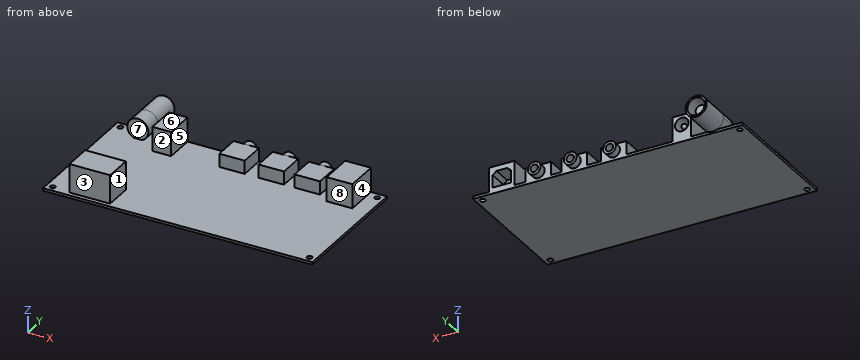
from build123d import *

# Parameters (mm, degrees)
F0_W           = 127
F0_H           = 63
F1_DEPTH       = 1.2
F2_R           = 1.25
F3_DEPTH       = 1.2
F4_W           = 12
F4_H           = 12.13
F5_DEPTH       = 6.25
F6_R           = 3
F7_DEPTH       = 3.52
F8_R           = 1.775
F9_DEPTH       = 14
F10_W          = 12.12
F10_H          = 15.7
F11_DEPTH      = 11.43
F13_DEPTH      = 9
F14_W          = 8.84
F14_H          = 13.9
F15_DEPTH      = 11.4
F16_R          = 3.2
F17_DEPTH      = 9.25
F18_R          = 1.15
F19_DEPTH      = 8.25
F20_R          = 1
F21_R          = 5
F22_DEPTH      = 14
F22_DEPTH_BACK = 8
F23_R          = 4.1
F24_DEPTH      = 8.6
F25_R          = 2.3
F26_DEPTH      = 4.9
F27_W          = 19.16
F27_H          = 13.3
F28_DEPTH      = 13.46


with BuildPart() as f1:
    # F0 (on Top) → F1 (new body)
    with BuildSketch(Plane.XY):
        with Locations((63.5, -31.5)):
            Rectangle(F0_W, F0_H)
    extrude(amount=F1_DEPTH)

    # F2 (on face) → F3 (cut, through all)
    with BuildSketch(Plane.XY.offset(1.2)):
        with Locations((2.955, -2.955)):
            Circle(F2_R)
        with Locations((2.955, -60.045)):
            Circle(F2_R)
        with Locations((124.045, -60.045)):
            Circle(F2_R)
        with Locations((124.045, -2.955)):
            Circle(F2_R)
    extrude(amount=-F3_DEPTH, mode=Mode.SUBTRACT)

    # F4 (on face) → F5 (join)
    with BuildSketch(Plane.XY.offset(1.2)):
        with Locations((96.19, -6.065)):
            Rectangle(F4_W, F4_H)
        with Locations((79.2, -6.065)):
            Rectangle(F4_W, F4_H)
        with Locations((60.7, -6.065)):
            Rectangle(F4_W, F4_H)
    extrude(amount=F5_DEPTH)

    # F6 (on face) → F7 (join)
    with BuildSketch(Plane(origin=(0, 0, 0), x_dir=(-1, 0, 0), z_dir=(0, 1, 0))):
        with Locations((-96.19, 4.325)):
            Circle(F6_R)
        with Locations((-79.2, 4.325)):
            Circle(F6_R)
        with Locations((-60.7, 4.325)):
            Circle(F6_R)
    extrude(amount=F7_DEPTH)

    # F8 (on face) → F9 (cut)
    with BuildSketch(Plane(origin=(0, 3.52, 0), x_dir=(-1, 0, 0), z_dir=(0, 1, 0))):
        with Locations((-96.19, 4.325)):
            Circle(F8_R)
        with Locations((-79.2, 4.325)):
            Circle(F8_R)
        with Locations((-60.7, 4.325)):
            Circle(F8_R)
    extrude(amount=-F9_DEPTH, mode=Mode.SUBTRACT)

    # F10 (on face) → F11 (join)
    with BuildSketch(Plane.XY.offset(1.2)):
        with Locations((113.39, -7.85)):
            Rectangle(F10_W, F10_H)
    extrude(amount=F11_DEPTH)

    # F12 (on face) → F13 (cut)
    with BuildSketch(Plane(origin=(0, 0, 0), x_dir=(-1, 0, 0), z_dir=(0, 1, 0))):
        Polygon((-117.78, 8.72), (-117.78, 2.8), (-109, 2.8), (-109, 8.72), (-110.89, 10.2), (-115.89, 10.2), align=None)
    extrude(amount=-F13_DEPTH, mode=Mode.SUBTRACT)

    # F14 (on face) → F15 (join)
    with BuildSketch(Plane.XY.offset(1.2)):
        with Locations((28.58, -6.95)):
            Rectangle(F14_W, F14_H)
    extrude(amount=F15_DEPTH)

    # F16 (on face) → F17 (cut)
    with BuildSketch(Plane(origin=(0, 0, 0), x_dir=(-1, 0, 0), z_dir=(0, 1, 0))):
        with Locations((-28.58, 8.1)):
            Circle(F16_R)
    extrude(amount=-F17_DEPTH, mode=Mode.SUBTRACT)

    # F18 (on face) → F19 (join, through all)
    with BuildSketch(Plane(origin=(0, -9.25, 0), x_dir=(-1, 0, 0), z_dir=(0, 1, 0))):
        with Locations((-28.58, 8.1)):
            Circle(F18_R)
    extrude(amount=F19_DEPTH)

    # F20
    f20_edges = [f1.edges().sort_by_distance(p)[0] for p in [
        (29.73, -1, 8.1),
    ]]
    fillet(f20_edges, radius=F20_R)

    # F21 (on face) → F22 (join, two sides)
    with BuildSketch(Plane(origin=(0, 0, 0), x_dir=(-1, 0, 0), z_dir=(0, 1, 0))) as f22_sk:
        with Locations((-14, 5.77)):
            Circle(F21_R)
    extrude(amount=F22_DEPTH)
    extrude(f22_sk.sketch, amount=-F22_DEPTH_BACK)

    # F23 (on face) → F24 (cut)
    with BuildSketch(Plane(origin=(0, 14, 0), x_dir=(-1, 0, 0), z_dir=(0, 1, 0))):
        with Locations((-14, 5.77)):
            Circle(F23_R)
    extrude(amount=-F24_DEPTH, mode=Mode.SUBTRACT)

    # F25 (on face) → F26 (join, through all)
    with BuildSketch(Plane(origin=(0, 5.4, 0), x_dir=(-1, 0, 0), z_dir=(0, 1, 0))):
        with Locations((-14, 5.77)):
            Circle(F25_R)
    extrude(amount=F26_DEPTH)

    # F27 (on face) → F28 (join)
    with BuildSketch(Plane.XY.offset(1.2)):
        with Locations((20.88, -54.24)):
            Rectangle(F27_W, F27_H)
    extrude(amount=F28_DEPTH)


solid = f1.part
The listing builds one solid part. Answer for the finished solid, in the listing's coordinates (mm). Face numbers are marked on the shaded views. A direction names the side the tool comes from. Coordinates: 2 decimals unless noted, no trailing zeros. Write each loop counter-clockwise with the first axis right and the second up, starting at its lowest first coordinate (ties: lowest second). Pieces come first, ordered by that corner, then holes. Notation, with made-up numbers: M -13.75,73.25 L 4.25,73.25 A17 ccw 4.25,99.25 Z; hole C -22,15 d4. An arc over 180 degrees is marked long. Put each result on its own line as item: value. Start each with the question number.
1. A cutting plane is placed at C-C on x = 79.2. Write down the section's boundary in (y, z) (3 decimals).
2. A cutting plane is placed at A-A on y = -54. Write down the section's boundary in (x, z), then the cut area to 3 significant figures.
3. For a pull along Y with two mould halves and no side action, classify the marked faces 6, 7 and 8 as pulls with the +Y half, pulls with the -Y half, needs draft (parallel to the pull), parting line crosses it, or undercut.
4. A cutting plane is placed at B-B on x = 14. Write down the section's boundary in (y, z), then the cut area to 3 significant figures.
5. Which of the six approach directions +Z, -Z, +X, -X, +Y, -Y give full straight-line access (tool end or side, diameter ignored) to the marked faces 1, 2, 3, 4 and 5?
6. Consider line 1 (Z direction, x = 14, y = 8); line 2 (X direction, y = -7, z = 1.25); line 3 (Z direction, x = 96, y = -3). Determine where each line is inside the solid, lowest interval first. Write a range as from..to.
7. A cutting plane is placed at D-D on y = -40.5. Write down the section's boundary in (x, z).
8. Flat-ended cylindrical pins translate along their axes: P1, Ø1.9, axis at x = 58.5, z = 3.5, coming from the -Y side; P2, Ø8, axis at x = 50.5, z = 2.5, coming from the +Y side; P3, Ø1.8, axis at x = 80, z = 3.5, coming from the +Y side. Find the tip coordinate at first contact, or state that the pin passes through.
Resolved:
1. outline: M -63,0 L 0,0 L 0,1.325 L 3.52,1.325 L 3.52,2.55 L -10.48,2.55 L -10.48,6.1 L 3.52,6.1 L 3.52,7.325 L 0,7.325 L 0,7.45 L -12.13,7.45 L -12.13,1.2 L -63,1.2 Z
2. outline: M 0,0 L 127,0 L 127,1.2 L 30.46,1.2 L 30.46,14.66 L 11.3,14.66 L 11.3,1.2 L 0,1.2 Z
2. area: 410 mm2
3. face 6: needs draft
3. face 7: undercut
3. face 8: pulls with the -Y half
4. outline: M -63,0 L 0,0 L 0,0.77 L 14,0.77 L 14,1.67 L 5.4,1.67 L 5.4,3.47 L 10.3,3.47 L 10.3,8.07 L 5.4,8.07 L 5.4,9.87 L 14,9.87 L 14,10.77 L -8,10.77 L -8,1.2 L -47.59,1.2 L -47.59,14.66 L -60.89,14.66 L -60.89,1.2 L -63,1.2 Z
4. area: 423 mm2
5. face 1: +Z, +X, -Y
5. face 2: +Z, -X
5. face 3: +Z, +X, -X, -Y
5. face 4: +Z, +X, +Y, -Y
5. face 5: +Z, +Y, -Y
6. line 1: z = 0.77..1.67, 3.47..8.07, 9.87..10.77
6. line 2: x = 11.86..16.14, 24.16..33, 54.7..66.7, 73.2..85.2, 90.19..102.19, 107.33..119.45
6. line 3: z = 0..2.56, 6.09..7.45
7. outline: M 0,0 L 127,0 L 127,1.2 L 0,1.2 Z
8. P1: stops at y = -12.13
8. P2: stops at y = 0
8. P3: stops at y = 3.52
